Input: dimensioned drawing with shaded views. Units: mm. Origin: part minimum x, y, z. A direction names the side the tool comes from. Coordinates: 2 decimals unless noted, no trailing zeros. Order: outer loops, then holes, each group sorted by start corner. A loop starts at its lowest first (then second) coordinate and runs counter-clockwise, first axis right, second up. Notation, with made-up numbers: (19.5, -34.75) -> (75.5, -34.75) arc R20 ccw to (75.5, -18.75) -> close; hole circle Ø5 at (-25, -21.5). An arc over 180 degrees is marked (long way). Put each result on its own line as item: value.
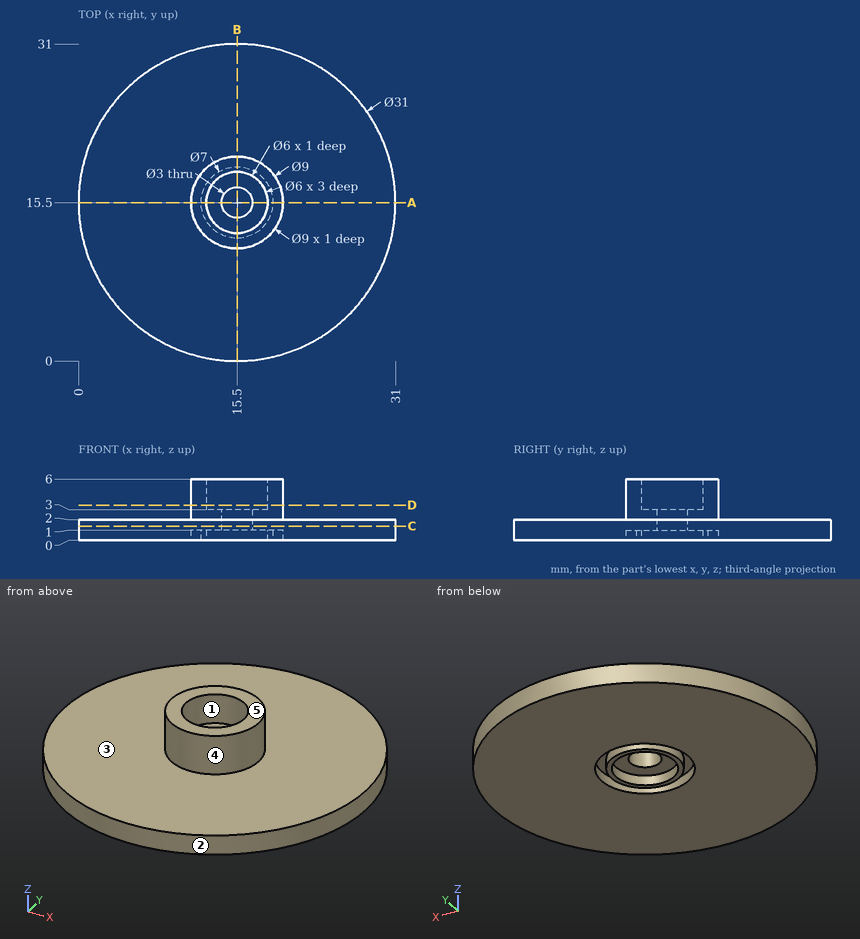
1. Pull-direction query (Y, two-part tool) for the marked faces 1, 2 and 3; classes: pulls with the +Y half, pulls with the -Y half, needs draft (parallel to the pull), parting line crosses it, or undercut.
Numbers:
face 1: undercut
face 2: parting line crosses it
face 3: needs draft
2. Cut plane C-C on z = 1.4. Output: boundary loops of the cut face in (x, y).
Numbers:
outline: circle Ø31 at (15.5, 15.5); hole circle Ø3 at (15.5, 15.5)
3. First-contact query: pin 1 (2.5 mm diameter, centred on x = 15.5, y = 15.5, fed in from -Z); pin 2 (1.8 mm diameter, centred on x = 15.5, y = 16.5, fed in from -Z); pin 3 (3 mm diameter, centred on x = 16, y = 15.5, fed in from +Z); pin 4 (3 mm diameter, centred on x = 18, z = 5, fed in from +Y). Flat tips, straight axial feed; report the tip coordinate or a pass-through.
Numbers:
pin 1: passes through
pin 2: stops at z = 1
pin 3: stops at z = 3
pin 4: stops at y = 19.89
4. Cut plane A-A on y = 15.5. Output: boundary loops of the cut face in (x, z), plus the area to 3 significant figures.
Numbers:
outline: (0, 0) -> (11, 0) -> (11, 1) -> (12, 1) -> (12, 0) -> (12.5, 0) -> (12.5, 1) -> (14, 1) -> (14, 3) -> (12.5, 3) -> (12.5, 6) -> (11, 6) -> (11, 2) -> (0, 2) -> close; (17, 1) -> (18.5, 1) -> (18.5, 0) -> (19, 0) -> (19, 1) -> (20, 1) -> (20, 0) -> (31, 0) -> (31, 2) -> (20, 2) -> (20, 6) -> (18.5, 6) -> (18.5, 3) -> (17, 3) -> close
area: 66.0 mm2
5. Ray query, line 1 along Y through (x, z) = (15.5, 0.35); line 2 along Y through (x, z) = (15.5, 1.55); line 3 along Y through (x, z) = (15.5, 4). Return the intervals inside material, ascending.
Numbers:
line 1: y = 0 to 11, 12 to 12.5, 18.5 to 19, 20 to 31
line 2: y = 0 to 14, 17 to 31
line 3: y = 11 to 12.5, 18.5 to 20
6. Set-up query: the marked faces 4 and 5. Return all of +Z, -Z, +X, -X, +Y, -Y with unobstructed straight access to the full face (end or side cutting, diameter ignored); none if empty.
Numbers:
face 4: +Z
face 5: +Z, +X, -X, +Y, -Y
7. Cut plane D-D on z = 3.45. Output: boundary loops of the cut face in (x, y), plus the area to 3 significant figures.
Numbers:
outline: circle Ø9 at (15.5, 15.5); hole circle Ø6 at (15.5, 15.5)
area: 35.3 mm2
